Can you work these out from the model? Positions are in its coordinate system, mm. A direction names the side the tool comes from. Round coordinates to 2 decimals unless told otherwise and drop trailing zeros. Loops run counter-clockwise (first coordinate to the right, second up) from the corner with the lowest first, then second, coordinate; pieces in that order, holes last. Notation, with made-up numbers: (82, -10.5) -> (98, -10.5) arc R22 cw to (98, 18.5) -> close; hole circle Ø5 at (41.25, -28). An arc over 180 degrees is marked (long way). Use a Markdown table: item, result.
from build123d import *

# Parameters (mm, degrees)
F1_DEPTH = 50.8
F2_T     = -12.7
F3_W     = 25.4
F3_H     = 38.1000075253
F4_DEPTH = 146.05
F5_DEPTH = 146.05


with BuildPart() as f1:
    # F0 (on Front) → F1 (new body)
    with BuildSketch(Plane.XZ):
        with BuildLine():
            Line((152.4, -150.9333811935), (152.4, 150.9333811935))
            Line((152.4, 150.9333811935), (85.725, 150.9333811935))
            Line((85.725, 150.9333811935), (85.725, 0))
            ThreePointArc((85.725, 0), (0, -85.725), (-85.725, 0))
            Line((-85.725, 0), (-85.725, 150.9333811935))
            Line((-85.725, 150.9333811935), (-152.4, 150.9333811935))
            Line((-152.4, 150.9333811935), (-152.4, -150.9333811935))
            Line((-152.4, -150.9333811935), (152.4, -150.9333811935))
        make_face()
    extrude(amount=F1_DEPTH)

    # F2
    f2_openings = [f1.faces().sort_by_distance(p)[0] for p in [
        (85.725, -25.4, 75.466691),
        (0, -25.4, -85.725),
        (-85.725, -25.4, 75.466691),
    ]]
    offset(amount=F2_T, openings=f2_openings)

    # F3 (on Right) → F4 (cut)
    with BuildSketch(Plane.YZ):
        with Locations((-25.1512676477, 151.2203067541)):
            Rectangle(F3_W, F3_H)
    extrude(amount=-F4_DEPTH, mode=Mode.SUBTRACT)

    # F3 (on Right) → F5 (cut)
    with BuildSketch(Plane.YZ):
        with Locations((-25.1512676477, 151.2203067541)):
            Rectangle(F3_W, F3_H)
    extrude(amount=F5_DEPTH, mode=Mode.SUBTRACT)


solid = f1.part
1. I want a section at D-D (y = -30). Please give me the cut outline in (x, z).
Answer sheet:
| item | result |
|---|---|
| outline | (-152.4, -150.93) -> (152.4, -150.93) -> (152.4, 150.93) -> (146.05, 150.93) -> (146.05, 132.17) -> (139.7, 132.17) -> (139.7, -138.23) -> (-139.7, -138.23) -> (-139.7, 132.17) -> (-146.05, 132.17) -> (-146.05, 150.93) -> (-152.4, 150.93) -> close |
2. I want a section at A-A (z = -91.5). Please give me the cut outline in (x, y).
Answer sheet:
| item | result |
|---|---|
| outline | (-152.4, -50.8) -> (152.4, -50.8) -> (152.4, 0) -> (-152.4, 0) -> close; hole (-139.7, -38.1) -> (139.7, -38.1) -> (139.7, -12.7) -> (-139.7, -12.7) -> close |
3. Which directions (+Z, -Z, +X, -X, +Y, -Y) give clear straight access to the entire face, cutting with the end or side of a thin tool? Please do faces 4 (the flat face through (152.4, -25, -2)), 5 (the flat face through (-146.05, -25, 142)), 6 (the flat face through (85.725, -44, 77)).
Answer sheet:
| item | result |
|---|---|
| face 4 | +Z, -Z, +X, +Y, -Y |
| face 5 | +Z |
| face 6 | +Z, +Y, -Y |
4. I want a section at C-C (z = 31.5). Please give me the cut outline in (x, y) (3 decimals), plus the area to 3 significant figures.
Answer sheet:
| item | result |
|---|---|
| outline | (-152.4, -50.8) -> (-85.725, -50.8) -> (-85.725, -38.1) -> (-139.7, -38.1) -> (-139.7, -12.7) -> (-85.725, -12.7) -> (-85.725, 0) -> (-152.4, 0) -> close; (85.725, -50.8) -> (152.4, -50.8) -> (152.4, 0) -> (85.725, 0) -> (85.725, -12.7) -> (139.7, -12.7) -> (139.7, -38.1) -> (85.725, -38.1) -> close |
| area | 4,030 mm² |
5. If we mould it in two halves opening along Y, with no side actions, what happens to faces 1 (the cylindrical face through (1.885, -6.261, -85.704)), 2 (the flat face through (-115, -37.851, 144)), 3 (the flat face through (-2, 0, -99))? For each: +Y half, -Y half, draft (parallel to the pull), parting line (faces both ways), or undercut.
Answer sheet:
| item | result |
|---|---|
| face 1 | draft |
| face 2 | undercut |
| face 3 | +Y half |
6. I want a section at B-B (x = 91). Please give me the cut outline in (y, z).
Answer sheet:
| item | result |
|---|---|
| outline | (-50.8, -150.93) -> (0, -150.93) -> (0, 150.93) -> (-12.45, 150.93) -> (-12.45, 132.17) -> (-12.7, 132.17) -> (-12.7, -138.23) -> (-38.1, -138.23) -> (-38.1, 138.23) -> (-37.85, 138.23) -> (-37.85, 150.93) -> (-50.8, 150.93) -> close |
7. Will these pins go through, and if not, where does the flat tip stop? pin 1 Ø20.5 at (x, y) = (-53.5, -30.5) entering from +Z; pin 2 Ø7.5 at (x, y) = (111, -19) entering from +Z.
Answer sheet:
| item | result |
|---|---|
| pin 1 | stops at z = -60.85 |
| pin 2 | stops at z = -138.23 |
8. I need wall thicknesses on line 1 (Y direction, x = -101.5, z = -13); line 2 (X direction, y = -47, z = 80) (3 decimals); line 3 (X direction, y = -29.5, z = -118). Which ranges of each line are inside material? Lowest first, please.
Answer sheet:
| item | result |
|---|---|
| line 1 | y = -50.8 to -38.1, -12.7 to 0 |
| line 2 | x = -152.4 to -85.725, 85.725 to 152.4 |
| line 3 | x = -152.4 to -139.7, 139.7 to 152.4 |
